For this review, take the finished solid that the model builds, in its own axes (mm). Round coordinates to 2 decimals unless told otherwise and drop trailing zeros. Write each loop counter-clockwise with the first axis right and the second up, starting at its lowest first coordinate (ties: lowest second). Pieces come first, ordered by that corner, then holes.
from build123d import *

# Parameters (mm, degrees)
SKETCH_219_R           = 1.45
SKETCH_219_R_2         = 1.7
EXTRUDE_2_DEPTH        = 2
CUT_EXTRUDE_641_DEPTH  = 61.860496219
CUT_EXTRUDE_1124_DEPTH = 61.860496219
CHAMFER_C0_2_SIZE      = 0.2
CUT_EXTRUDE_2015_DEPTH = 61.860496219
SKETCH_M3_R            = 1.7
CUT_EXTRUDE_2116_DEPTH = 61.860496219


with BuildPart() as part:
    # Sketch 219 → 屏幕承架厚2 (new body)
    with BuildSketch(Plane.XY):
        with BuildLine():
            Line((-24, -42), (24, -42))
            ThreePointArc((24, -42), (38.142135624, -36.142135624), (44, -22))
            Line((44, -22), (44, 22))
            ThreePointArc((44, 22), (38.142135624, 36.142135624), (24, 42))
            Line((24, 42), (-24, 42))
            ThreePointArc((-24, 42), (-38.142135624, 36.142135624), (-44, 22))
            Line((-44, 22), (-44, -22))
            ThreePointArc((-44, -22), (-38.142135624, -36.142135624), (-24, -42))
        make_face()
        with Locations((-29.35, 8.45)):
            Circle(SKETCH_219_R, mode=Mode.SUBTRACT)
        with Locations((-29.35, -32.45)):
            Circle(SKETCH_219_R, mode=Mode.SUBTRACT)
        with Locations((30.12, 8.45)):
            Circle(SKETCH_219_R, mode=Mode.SUBTRACT)
        with Locations((30.12, -32.45)):
            Circle(SKETCH_219_R, mode=Mode.SUBTRACT)
        with Locations((-39, -28)):
            Circle(SKETCH_219_R_2, mode=Mode.SUBTRACT)
        with Locations((-39, 28)):
            Circle(SKETCH_219_R_2, mode=Mode.SUBTRACT)
        with Locations((39, -28)):
            Circle(SKETCH_219_R_2, mode=Mode.SUBTRACT)
        with Locations((39, 28)):
            Circle(SKETCH_219_R_2, mode=Mode.SUBTRACT)
        with BuildLine():
            Line((-21, -28), (21, -28))
            ThreePointArc((21, -28), (23.828427125, -26.828427125), (25, -24))
            Line((25, -24), (25, 0))
            ThreePointArc((25, 0), (23.828427125, 2.828427125), (21, 4))
            Line((21, 4), (-21, 4))
            ThreePointArc((-21, 4), (-23.828427125, 2.828427125), (-25, 0))
            Line((-25, 0), (-25, -24))
            ThreePointArc((-25, -24), (-23.828427125, -26.828427125), (-21, -28))
        make_face(mode=Mode.SUBTRACT)
    extrude(amount=EXTRUDE_2_DEPTH)

    # 摄像板可换安装区26乘25 → Cut-Extrude 641 (cut, through all)
    with BuildSketch(Plane.XY):
        with BuildLine():
            Line((-11, 17.5), (11, 17.5))
            ThreePointArc((11, 17.5), (12.414213562, 18.085786438), (13, 19.5))
            Line((13, 19.5), (13, 40.5))
            ThreePointArc((13, 40.5), (12.414213562, 41.914213562), (11, 42.5))
            Line((11, 42.5), (-11, 42.5))
            ThreePointArc((-11, 42.5), (-12.414213562, 41.914213562), (-13, 40.5))
            Line((-13, 40.5), (-13, 19.5))
            ThreePointArc((-13, 19.5), (-12.414213562, 18.085786438), (-11, 17.5))
        make_face()
    extrude(amount=CUT_EXTRUDE_641_DEPTH, mode=Mode.SUBTRACT)

    # Sketch 697 → Cut-Extrude 1124 (cut, through all)
    with BuildSketch(Plane.XY):
        with BuildLine():
            Line((-38.25, -21), (-37.75, -21))
            ThreePointArc((-37.75, -21), (-37.042893219, -20.707106781), (-36.75, -20))
            Line((-36.75, -20), (-36.75, -12))
            ThreePointArc((-36.75, -12), (-37.042893219, -11.292893219), (-37.75, -11))
            Line((-37.75, -11), (-38.25, -11))
            ThreePointArc((-38.25, -11), (-38.957106781, -11.292893219), (-39.25, -12))
            Line((-39.25, -12), (-39.25, -20))
            ThreePointArc((-39.25, -20), (-38.957106781, -20.707106781), (-38.25, -21))
        make_face()
        with BuildLine():
            Line((-38.25, -5), (-37.75, -5))
            ThreePointArc((-37.75, -5), (-37.042893219, -4.707106781), (-36.75, -4))
            Line((-36.75, -4), (-36.75, 4))
            ThreePointArc((-36.75, 4), (-37.042893219, 4.707106781), (-37.75, 5))
            Line((-37.75, 5), (-38.25, 5))
            ThreePointArc((-38.25, 5), (-38.957106781, 4.707106781), (-39.25, 4))
            Line((-39.25, 4), (-39.25, -4))
            ThreePointArc((-39.25, -4), (-38.957106781, -4.707106781), (-38.25, -5))
        make_face()
        with BuildLine():
            Line((37.75, -21), (38.25, -21))
            ThreePointArc((38.25, -21), (38.957106781, -20.707106781), (39.25, -20))
            Line((39.25, -20), (39.25, -12))
            ThreePointArc((39.25, -12), (38.957106781, -11.292893219), (38.25, -11))
            Line((38.25, -11), (37.75, -11))
            ThreePointArc((37.75, -11), (37.042893219, -11.292893219), (36.75, -12))
            Line((36.75, -12), (36.75, -20))
            ThreePointArc((36.75, -20), (37.042893219, -20.707106781), (37.75, -21))
        make_face()
        with BuildLine():
            Line((37.75, -5), (38.25, -5))
            ThreePointArc((38.25, -5), (38.957106781, -4.707106781), (39.25, -4))
            Line((39.25, -4), (39.25, 4))
            ThreePointArc((39.25, 4), (38.957106781, 4.707106781), (38.25, 5))
            Line((38.25, 5), (37.75, 5))
            ThreePointArc((37.75, 5), (37.042893219, 4.707106781), (36.75, 4))
            Line((36.75, 4), (36.75, -4))
            ThreePointArc((36.75, -4), (37.042893219, -4.707106781), (37.75, -5))
        make_face()
    extrude(amount=CUT_EXTRUDE_1124_DEPTH, mode=Mode.SUBTRACT)

    # 非功能外缘倒角_C0.2
    chamfer_c0_2_edges = [part.edges().sort_by_distance(p)[0] for p in [
        (38.142135624, -36.142135624, 2),
        (-38.957106781, -4.707106781, 2),
        (-38, -5, 2),
        (-37.042893219, -4.707106781, 2),
        (-36.75, 0, 2),
        (-37.042893219, 4.707106781, 2),
        (-38, 5, 2),
        (-38.957106781, 4.707106781, 2),
        (-39.25, 0, 2),
        (37.042893219, -20.707106781, 2),
        (38, -21, 2),
        (38.957106781, -20.707106781, 2),
        (39.25, -16, 2),
        (38.957106781, -11.292893219, 2),
        (38, -11, 2),
        (37.042893219, -11.292893219, 2),
        (36.75, -16, 2),
        (44, 0, 2),
        (37.042893219, -4.707106781, 2),
        (38, -5, 2),
        (38.957106781, -4.707106781, 2),
        (39.25, 0, 2),
        (38.957106781, 4.707106781, 2),
        (38, 5, 2),
        (37.042893219, 4.707106781, 2),
        (36.75, 0, 2),
        (-38.957106781, -20.707106781, 2),
        (-38, -21, 2),
        (-37.042893219, -20.707106781, 2),
        (-36.75, -16, 2),
        (-37.042893219, -11.292893219, 2),
        (-38, -11, 2),
        (-38.957106781, -11.292893219, 2),
        (-39.25, -16, 2),
        (38.142135624, 36.142135624, 2),
        (18.161437828, 42, 2),
        (-38.142135624, 36.142135624, 2),
        (-23.828427125, -26.828427125, 2),
        (0, -28, 2),
        (23.828427125, -26.828427125, 2),
        (25, -12, 2),
        (23.828427125, 2.828427125, 2),
        (0, 4, 2),
        (-23.828427125, 2.828427125, 2),
        (-44, 0, 2),
        (-25, -12, 2),
        (-38.142135624, -36.142135624, 2),
        (-18.161437828, 42, 2),
        (0, -42, 2),
        (12.822875656, 41.322875656, 2),
        (-12.822875656, 41.322875656, 2),
        (-13, 30, 2),
        (-12.414213562, 18.085786438, 2),
        (0, 17.5, 2),
        (12.414213562, 18.085786438, 2),
        (13, 30, 2),
    ]]
    chamfer(chamfer_c0_2_edges, length=CHAMFER_C0_2_SIZE)

    # 相机螺母与后插座避空28乘29_5 → Cut-Extrude 2015 (cut, through all)
    with BuildSketch(Plane.XY):
        with BuildLine():
            Line((-12, 13), (12, 13))
            ThreePointArc((12, 13), (13.414213562, 13.585786438), (14, 15))
            Line((14, 15), (14, 40.5))
            ThreePointArc((14, 40.5), (13.414213562, 41.914213562), (12, 42.5))
            Line((12, 42.5), (-12, 42.5))
            ThreePointArc((-12, 42.5), (-13.414213562, 41.914213562), (-14, 40.5))
            Line((-14, 40.5), (-14, 15))
            ThreePointArc((-14, 15), (-13.414213562, 13.585786438), (-12, 13))
        make_face()
    extrude(amount=CUT_EXTRUDE_2015_DEPTH, mode=Mode.SUBTRACT)

    # 相机托架双M3连接孔 → Cut-Extrude 2116 (cut, through all)
    with BuildSketch(Plane.XY):
        with Locations((-20, 25)):
            Circle(SKETCH_M3_R)
        with Locations((20, 25)):
            Circle(SKETCH_M3_R)
    extrude(amount=CUT_EXTRUDE_2116_DEPTH, mode=Mode.SUBTRACT)


solid = part.part
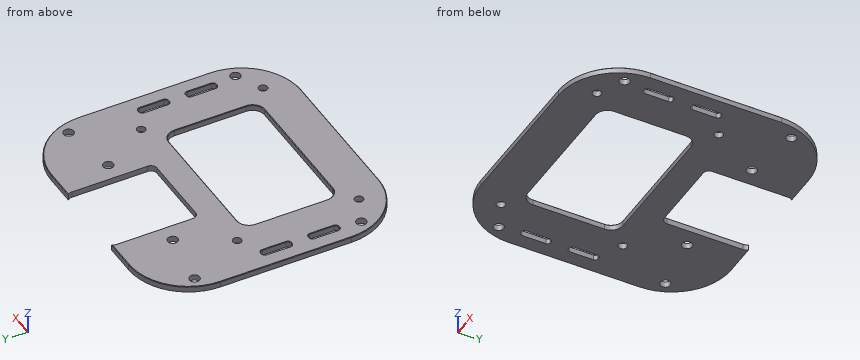
(1) We need section A-A, the plane x = 20. Give the boundary of the cut face in (y, z).
Geometry check:
outline: (-42, 0) - (-28, 0) - (-28, 1.8) - (-28.2, 2) - (-41.8, 2) - (-42, 1.8) - close; (4, 0) - (23.3, 0) - (23.3, 2) - (4.2, 2) - (4, 1.8) - close; (26.7, 0) - (42, 0) - (42, 1.8) - (41.8, 2) - (26.7, 2) - close
(2) We need section D-D, the plane z = 0.95. State how many separate pieces and enclosed holes the cut face has, and give its area (3 significant figures).
Geometry check:
separate pieces: 1
enclosed holes: 15
area: 4,480 mm2
(3) We need section C-C, the plane x = -1.5. Give the boundary of the cut face in (y, z).
Geometry check:
outline: (-42, 0) - (-28, 0) - (-28, 1.8) - (-28.2, 2) - (-41.8, 2) - (-42, 1.8) - close; (4, 0) - (13, 0) - (13, 2) - (4.2, 2) - (4, 1.8) - close
(4) For line 1 along Y through (x, z) = (-20, 0.7); line 2 along X through (y, z) = (-12.5, 0.7); line 3 along Y through (x, z) = (-6, 1.7), list the stretches that pass through material, from the lowest coordinate up.
Geometry check:
line 1: y = -42 to -28, 4 to 23.3, 26.7 to 42
line 2: x = -44 to -39.25, -36.75 to -25, 25 to 36.75, 39.25 to 44
line 3: y = -42 to -28, 4 to 13
(5) We need section B-B, the plane y = -8. Give the boundary of the cut face in (x, z), and give its area (3 significant figures).
Geometry check:
outline: (-44, 0) - (-25, 0) - (-25, 1.8) - (-25.2, 2) - (-43.8, 2) - (-44, 1.8) - close; (25, 0) - (44, 0) - (44, 1.8) - (43.8, 2) - (25.2, 2) - (25, 1.8) - close
area: 75.9 mm2
(6) For pin 1 Ø0.6 at (x, z) = (-38, 0.5) entering from +Y, flat-tipped, find the tip position at first contact; note if it passes through.
Geometry check:
pin 1: stops at y = 36.57
